Geometry check sheet. Reference: the model listing, model coordinates, mm. A direction names the side the tool comes from. Round coordinates to 2 decimals unless told otherwise and drop trailing zeros. Write each loop counter-clockwise with the first axis right and the second up, starting at its lowest first coordinate (ties: lowest second). Pieces come first, ordered by that corner, then holes. Notation, with made-up numbers: M 19.25,0 L 71.25,0 A17 cw 71.25,27 Z; hole C -27,32 d2. An arc over 180 degrees is marked long. Put each result on its own line as item: value. Start each with the question number.
(1) Section check A-A on x = 5.08. Record the cut outline in (y, z) (3 decimals).
(2) Section check C-C on z = -24.5. Record the cut outline in (x, y) (3 decimals), then the cut area to 3 significant figures.
(3) Gauge pin test, flat ends, axial feed: pin 1 (1 mm diameter, centred on x = -7, z = -2.5, fed in from +Y) (3 decimals); pin 2 (3 mm diameter, centred on x = 6.5, z = -9, fed in from +Y); pin 3 (3 mm diameter, centred on x = -4, z = -4.5, fed in from +Y) (3 decimals); pin 4 (4 mm diameter, centred on x = -7, z = 3, fed in from -Y). Record the tip position at first contact, or that the pin passes through.
(4) Material ranges on probe 1 along Z at (x, y) = (5.08, 5.55) (3 decimals); probe 2 along Z at (x, y) = (5.08, 2.1) (3 decimals); probe 3 along Y at (x, z) = (1, 0), recorded low to high.
(5) Section check B-B on x = 8. Record the cut outline in (y, z) (3 decimals), then the cut area to 3 significant figures.
(6) Tool access check on faces 1 (the flat face through (-4, 15, 28.575)), 2 (the cylindrical face through (0.72, 5.14, 9.33)), 3 (the flat face through (6, 6.35, -3)). Record the directions out of +Z, -Z, +X, -X, +Y, -Y that give a thin tool (end or side, any length) a straight path to the whole face; none if there is none.
(7) Section check D-D on y = 7.5. Record the cut outline in (x, z) (3 decimals).
from build123d import *

# Parameters (mm, degrees)
SKETCH2_W                                      = 19.05
SKETCH2_H                                      = 57.15
BOSS_EXTRUDE2_DEPTH                            = 38.1
CUT_EXTRUDE2_DEPTH                             = 20.05
SKETCH7_W                                      = 25.4
SKETCH7_H                                      = 63.5
CUT_EXTRUDE5_DEPTH                             = 63.5
FILLET3_R                                      = 3.81
CBORE_FOR_8_BUTTON_HEAD_CAP_SCREW1_D           = 4.4958
CBORE_FOR_8_BUTTON_HEAD_CAP_SCREW1_CBORE_D     = 8.73252
CBORE_FOR_8_BUTTON_HEAD_CAP_SCREW1_CBORE_DEPTH = 2.4638
BOSS_EXTRUDE3_DEPTH                            = 1.016


with BuildPart() as part:
    # Sketch2 → Boss-Extrude2 (new body)
    with BuildSketch(Plane(origin=(0, 0, 0), x_dir=(1, 0, 0), z_dir=(0, 1, 0))):
        Rectangle(SKETCH2_W, SKETCH2_H)
    extrude(amount=BOSS_EXTRUDE2_DEPTH)

    # Sketch4 → Cut-Extrude2 (cut, through all)
    with BuildSketch(Plane(origin=(9.525, 0, 0), x_dir=(0, 0, -1), z_dir=(1, 0, 0))):
        Polygon((28.575, 0), (-9.525, 38.1), (28.575, 38.1), align=None)
    extrude(amount=-CUT_EXTRUDE2_DEPTH, mode=Mode.SUBTRACT)

    # Sketch7 → Cut-Extrude5 (cut)
    with BuildSketch(Plane.XY.offset(28.575)):
        with Locations((9.525, 38.1)):
            Rectangle(SKETCH7_W, SKETCH7_H)
    extrude(amount=-CUT_EXTRUDE5_DEPTH, mode=Mode.SUBTRACT)

    # Fillet3
    fillet3_edges = [part.edges().sort_by_distance(p)[0] for p in [
        (-3.175, 6.35, 3.175),
    ]]
    fillet(fillet3_edges, radius=FILLET3_R)

    # CBORE for #8 Button Head Cap Screw1 (through all)
    with Locations(Plane(origin=(0, 6.35, 0), x_dir=(1, 0, 0), z_dir=(0, 1, 0))):
        with Locations((5.08, -22.225), (5.08, -9.525)):
            CounterBoreHole(CBORE_FOR_8_BUTTON_HEAD_CAP_SCREW1_D / 2, CBORE_FOR_8_BUTTON_HEAD_CAP_SCREW1_CBORE_D / 2, CBORE_FOR_8_BUTTON_HEAD_CAP_SCREW1_CBORE_DEPTH)

    # Sketch12 → Boss-Extrude3 (add)
    with BuildSketch(Plane(origin=(9.525, 0, 0), x_dir=(0, 0, -1), z_dir=(1, 0, 0))):
        Polygon((28.575, 0), (22.225, 6.35), (-28.575, 6.35), (-28.575, 0), align=None)
    extrude(amount=BOSS_EXTRUDE3_DEPTH)


solid = part.part
Answers follow:
1. outline: M 0,-28.575 L 6.35,-22.225 L 6.35,5.159 L 3.886,5.159 L 3.886,7.277 L 0,7.277 Z; M 0,11.773 L 3.886,11.773 L 3.886,13.891 L 6.35,13.891 L 6.35,17.859 L 3.886,17.859 L 3.886,19.977 L 0,19.977 Z; M 0,24.473 L 3.886,24.473 L 3.886,26.591 L 6.35,26.591 L 6.35,28.575 L 0,28.575 Z
2. outline: M -9.525,0 L 10.541,0 L 10.541,4.075 L -9.525,4.075 Z
2. area: 81.8 mm^2
3. pin 1: stops at y = 26.575
3. pin 2: stops at y = 6.35
3. pin 3: stops at y = 25.575
3. pin 4: stops at y = 0
4. probe 1: z = -23.025 to 5.159, 13.891 to 17.859, 26.591 to 28.575
4. probe 2: z = -26.475 to 7.277, 11.773 to 19.977, 24.473 to 28.575
4. probe 3: y = 0 to 6.35
5. outline: M 0,-28.575 L 6.35,-22.225 L 6.35,6.279 L 3.886,6.279 L 3.886,12.771 L 6.35,12.771 L 6.35,18.979 L 3.886,18.979 L 3.886,25.471 L 6.35,25.471 L 6.35,28.575 L 0,28.575 Z
5. area: 311 mm^2
6. face 1: +Z, +X, -X, +Y, -Y
6. face 2: +Y
6. face 3: +Z, -Z, +X, +Y
7. outline: M -9.525,-21.075 L -2.093,-21.075 L -2.093,28.575 L -9.525,28.575 Z
